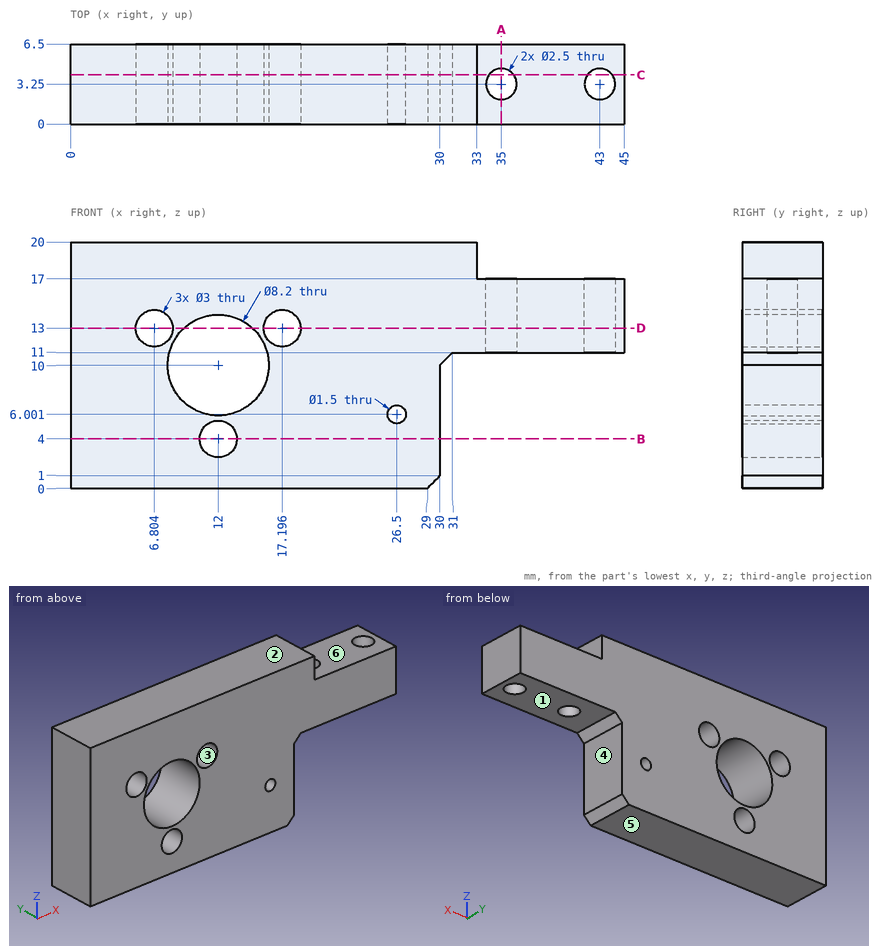
Check sheet for the drawn part. Datum: minimum x, y, z corner. Units: mm. A direction names the side the tool comes from. Round coordinates to 2 decimals unless told otherwise and drop trailing zeros. Order: outer loops, then holes, each group sorted by start corner. A loop starts at its lowest first (then second) coordinate and runs counter-clockwise, first axis right, second up. Notation, with made-up numbers: (66.5, 28) -> (114.5, 28) arc R23 ccw to (114.5, 42) -> close; hole circle Ø2 at (24, 75). An arc over 180 degrees is marked (long way). Return JSON: item names as keys, results as strings. Group by question number.
Q1. Section check C-C, the plane y = 4. Record the boundary of the cut face in (x, z), plus the area to 3 significant figures.
Q2. Tool access check on the marked faces 1 and 2. Record the directions out of +Z, -Z, +X, -X, +Y, -Y that give a thin tool (end or side, any length) a straight path to the whole face; none if there is none.
Q3. Section check D-D, the plane z = 13. Count the separate pieces of the cut face and the enclosed holes in it, plus the area to 3 significant figures.
Q4. Release check for a two-part mould opening along Z. For the marked faces 3, 4, 5 and 6 record: released by +Z, released by -Z, zero draft, split by the parting line, or undercut.
Q5. Material ranges on probe 1 along Y at (x, z) = (35, 13); probe 2 along Z at (x, y) = (11.5, 5) (1 decimal); probe 3 along X at (y, z) = (4.75, 4), recorded low to high. Write a range as from..to.
Q6. Section check B-B, the plane z = 4. Record the boundary of the cut face in (x, y), plus the area to 4 significant figures.
Q7. Section check A-A, the plane x = 35. Record the boundary of the cut face in (y, z), plus the area to 3 significant figures.
Q8. Gauge pin test, flat ends, axial feed: pin 1 (2 mm diameter, centred on x = 35, y = 3.25, fed in from +Z); pin 2 (3 mm diameter, centred on x = 38.5, y = 3.5, fed in from -Z); pin 3 (1.5 mm diameter, centred on y = 4.5, z = 18, fed in from +X). Record the tip position at first contact, or that the pin passes through.
Numbers:
{
 "1": {"outline": "(0, 0) -> (29, 0) -> (30, 1) -> (30, 10) -> (31, 11) -> (34, 11) -> (34, 17) -> (33, 17) -> (33, 20) -> (0, 20) -> close; (36, 11) -> (42, 11) -> (42, 17) -> (36, 17) -> close; (44, 11) -> (45, 11) -> (45, 17) -> (44, 17) -> close; hole circle Ø3 at (6.8, 13); hole circle Ø8.2 at (12, 10); hole circle Ø3 at (12, 4); hole circle Ø3 at (17.2, 13); hole circle Ø1.5 at (26.5, 6)", "area": "599 mm^2"},
 "2": {"face 1": "-Z, +X, +Y, -Y", "face 2": "+Z, +X, -X, +Y, -Y"},
 "3": {"separate pieces": "4", "enclosed holes": "2", "area": "207 mm^2"},
 "4": {"face 3": "undercut", "face 4": "zero draft", "face 5": "released by -Z", "face 6": "released by +Z"},
 "5": {"probe 1": "0..2, 4.5..6.5", "probe 2": "0..2.6, 5.4..5.9, 14.1..20", "probe 3": "0..10.5, 13.5..30"},
 "6": {"outline": "(0, 0) -> (10.5, 0) -> (10.5, 6.5) -> (0, 6.5) -> close; (13.5, 0) -> (30, 0) -> (30, 6.5) -> (13.5, 6.5) -> close", "area": "175.5 mm^2"},
 "7": {"outline": "(0, 11) -> (2, 11) -> (2, 17) -> (0, 17) -> close; (4.5, 11) -> (6.5, 11) -> (6.5, 17) -> (4.5, 17) -> close", "area": "24.0 mm^2"},
 "8": {"pin 1": "through", "pin 2": "z = 11", "pin 3": "x = 33"}
}
